```python
from build123d import *

# Parameters (mm, degrees)
ESQUISSE1_W             = 190
ESQUISSE1_H             = 46
ESQUISSE1_R             = 19.2
BOSS_EXTRU_1_DEPTH      = 4
ESQUISSE2_R             = 1.52
ENL_V_MAT_EXTRU_1_DEPTH = 5
CONG_2_R                = 1
CONG_3_R                = 0.5


with BuildPart() as part:
    # Esquisse1 → Boss.-Extru.1 (new body)
    with BuildSketch(Plane.XY):
        with Locations((66.068886156, 0)):
            Rectangle(ESQUISSE1_W, ESQUISSE1_H)
        Circle(ESQUISSE1_R, mode=Mode.SUBTRACT)
        with Locations((44.045924104, 0)):
            Circle(ESQUISSE1_R, mode=Mode.SUBTRACT)
        with Locations((88.091848208, 0)):
            Circle(ESQUISSE1_R, mode=Mode.SUBTRACT)
        with Locations((132.137772312, 0)):
            Circle(ESQUISSE1_R, mode=Mode.SUBTRACT)
    extrude(amount=BOSS_EXTRU_1_DEPTH)

    # Esquisse2 → Enlèv. mat.-Extru.1 (cut)
    with BuildSketch(Plane.XY.offset(4)):
        with Locations((-23.935283884, 17.499369506)):
            Circle(ESQUISSE2_R)
        with Locations(Location((-23.935283884, -17.499369506, 0), (0, 0, 180))):
            Circle(ESQUISSE2_R)
        with Locations((156.073056196, -17.499369506)):
            Circle(ESQUISSE2_R)
        with Locations(Location((156.073056196, 17.499369506, 0), (0, 0, 180))):
            Circle(ESQUISSE2_R)
    extrude(amount=-ENL_V_MAT_EXTRU_1_DEPTH, mode=Mode.SUBTRACT)

    # Congé2
    cong_2_edges = [part.edges().sort_by_distance(p)[0] for p in [
        (161.068886156, -23, 2),
        (-28.931113844, -23, 2),
        (-28.931113844, 23, 2),
        (161.068886156, 23, 2),
    ]]
    fillet(cong_2_edges, radius=CONG_2_R)

    # Congé3
    cong_3_edges = [part.edges().sort_by_distance(p)[0] for p in [
        (-19.2, 0, 4),
        (24.845924104, 0, 4),
        (68.891848208, 0, 4),
        (112.937772312, 0, 4),
    ]]
    fillet(cong_3_edges, radius=CONG_3_R)


solid = part.part
```
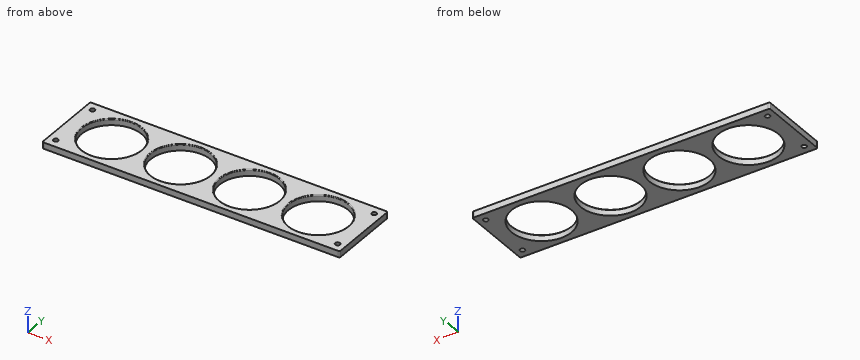
Check sheet for the modelled part. Datum: model origin and axes. Units: mm. Coordinates: 2 decimals unless noted, no trailing zeros. Order: outer loops, then holes, each group sorted by start corner. A loop starts at its lowest first (then second) coordinate and runs counter-clockwise, first axis right, second up. Notation, with made-up numbers: M 31.25,3 L 41.25,3 A13 ccw 41.25,20 Z; hole C 39,-35 d6. An arc over 180 degrees is marked long. One line per question, with ' | ' between items. Start each with the question number.
Item 1: Sectioned sample at B-B on x = 0. Record the cut outline in (y, z), and give its area (3 significant figures).
Item 2: Sectioned sample at C-C on z = 2.5. Count the separate pieces of the cut face and the enclosed holes in it, and give its area (3 significant figures).
Item 3: Material ranges on line 1 (X direction, y = 0.5, z = 2.3); line 2 (X direction, y = -11, z = 1.75); line 3 (Y direction, x = 0.5, z = 1.2), recorded low to high.
Item 4: Gauge pin test, flat ends, axial feed: P1, Ø2.5, axis at x = -23.94, y = -17.5, coming from the +Z side; P2, Ø5, axis at x = 156.07, y = -17.5, coming from the -Z side. Record the tip position at first contact, or that the pin passes through.
Item 5: Sectioned sample at A-A on y = 0. Record the cut outline in (x, z), and give its area (3 significant figures).
Answer below:
1) outline: M -23,0 L -19.2,0 L -19.2,3.5 A0.5 ccw -19.7,4 L -23,4 Z; M 19.2,0 L 23,0 L 23,4 L 19.7,4 A0.5 ccw 19.2,3.5 Z | area: 30.3 mm^2
2) separate pieces: 1 | enclosed holes: 8 | area: 4,080 mm^2
3) line 1: x = -28.93 to -19.19, 19.19 to 24.85, 63.24 to 68.9, 107.29 to 112.94, 151.33 to 161.07 | line 2: x = -28.93 to -15.74, 15.74 to 28.31, 59.78 to 72.36, 103.83 to 116.4, 147.87 to 161.07 | line 3: y = -23 to -19.19, 19.19 to 23
4) P1: passes through | P2: stops at z = 0
5) outline: M -28.93,0 L -19.2,0 L -19.2,3.5 A0.5 ccw -19.7,4 L -28.93,4 Z; M 19.2,0 L 24.85,0 L 24.85,3.5 A0.5 ccw 24.35,4 L 19.7,4 A0.5 ccw 19.2,3.5 Z; M 63.25,0 L 68.89,0 L 68.89,3.5 A0.5 ccw 68.39,4 L 63.75,4 A0.5 ccw 63.25,3.5 Z; M 107.29,0 L 112.94,0 L 112.94,3.5 A0.5 ccw 112.44,4 L 107.79,4 A0.5 ccw 107.29,3.5 Z; M 151.34,0 L 161.07,0 L 161.07,4 L 151.84,4 A0.5 ccw 151.34,3.5 Z | area: 145 mm^2
